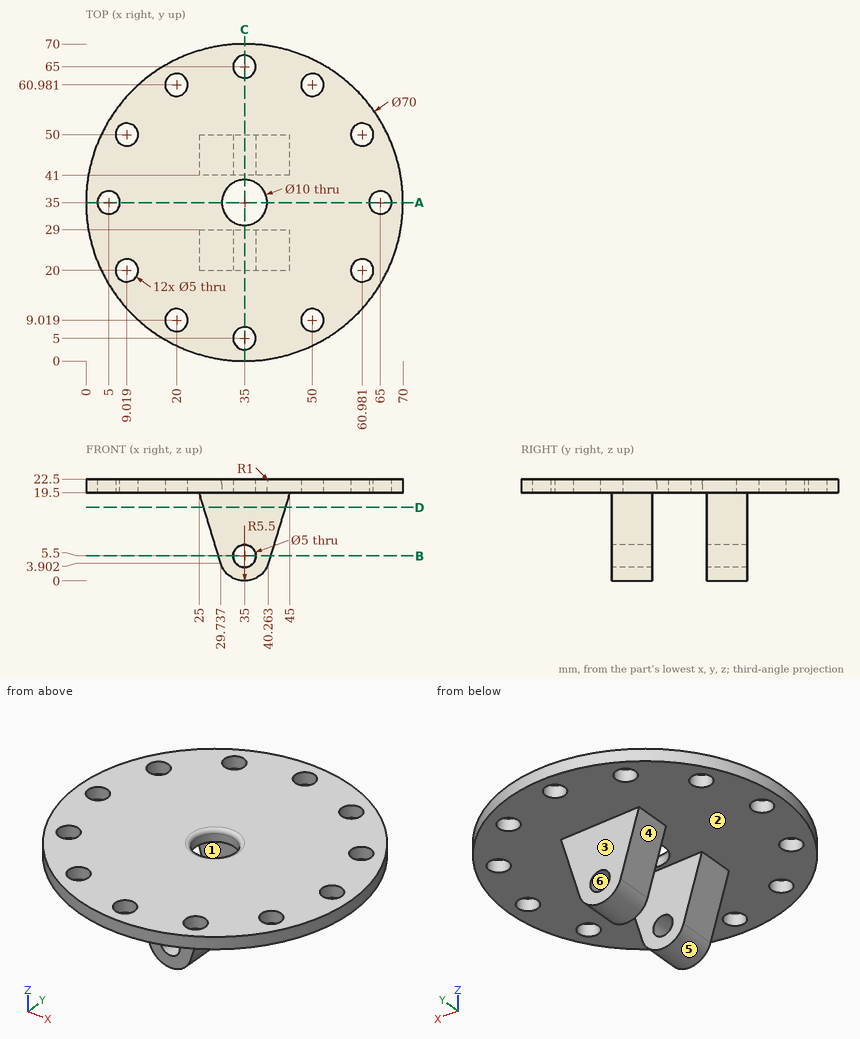
Study the drawing (mm; zero at the part's minimum x, y, z) and answer. A direction names the side the tool comes from. Give positions to 0.01 mm unless a question says otherwise; leave off trailing zeros. Write each loop counter-clockwise with the first axis right and the second up, starting at its lowest first coordinate (ties: lowest second). Pieces come first, ordered by that corner, then holes. Notation, with made-up numbers: (23.5, 3) - (48.5, 3) arc R18 cw to (48.5, 18) - close; hole circle Ø2 at (-17.5, 11.5). An arc over 180 degrees is marked (long way). Use CSV: the item, a comma, the result in double quotes. Start each with the question number.
(1) Given P1, Ø10, axis at x = 36, z = 7, coming from the +Y side; P2, Ø10, axis at x = 14, y = 62.5, coming from the -Z side; P3, Ø8, axis at x = 35, z = 5.5, coming from the -Y side; P4, Ø6, axis at x = 50, y = 9.02, coming from the +Z side, each flat-ended and moving along its own axis, determine where each tip first touches the part or whether it passes through.
(2) Find section B-B (z = 5.5). Give the vertices of the cut face in (x, y).
(3) Consider line 1 along Y through (x, z) = (35, 21.05); line 2 along Y through (x, z) = (34, 17); line 3 along Z through (x, y) = (36, 12). Determine where each line is inside the solid, lowest interval first.
(4) Find section D-D (z = 16.25). Give the vertices of the cut face in (x, y).
(5) For the marked faces 1, 2 and 3, determine the directions among +Z, -Z, +X, -X, +Y, -Y from which every point of the face is accessible in a straight line to the end or side of a thin tool.
(6) Find section A-A (y = 35). Give the vertices of the cut face in (x, z).
(7) Determine the mould class of the marked faces 4, 5 and 6 for opening direction X: +X half, -X half, draft (parallel to the pull), parting line (faces both ways), or undercut.
(8) Find section C-C (x = 35). Count the separate pieces of the cut face and the enclosed holes in it.
Findings below:
1,P1,"y = 50"
1,P2,"z = 19.5"
1,P3,"y = 20"
1,P4,"z = 22.5"
2,outline,"(29.25, 20) - (32.5, 20) - (32.5, 29) - (29.25, 29) - close; (29.25, 41) - (32.5, 41) - (32.5, 50) - (29.25, 50) - close; (37.5, 20) - (40.75, 20) - (40.75, 29) - (37.5, 29) - close; (37.5, 41) - (40.75, 41) - (40.75, 50) - (37.5, 50) - close"
3,line 1,"0 to 2.5, 7.5 to 30, 40 to 62.5, 67.5 to 70"
3,line 2,"20 to 29, 41 to 50"
3,line 3,"19.5 to 22.5"
4,outline,"(25.99, 20) - (44.01, 20) - (44.01, 29) - (25.99, 29) - close; (25.99, 41) - (44.01, 41) - (44.01, 50) - (25.99, 50) - close"
5,face 1,"-Z, +X, -X"
5,face 2,"-Z"
5,face 3,"-Z, +X, -X, +Y"
6,outline,"(0, 19.5) - (2.5, 19.5) - (2.5, 22.5) - (0, 22.5) - close; (7.5, 19.5) - (30, 19.5) - (30, 21.5) arc R1 ccw to (29, 22.5) - (7.5, 22.5) - close; (40, 19.5) - (62.5, 19.5) - (62.5, 22.5) - (41, 22.5) arc R1 ccw to (40, 21.5) - close; (67.5, 19.5) - (70, 19.5) - (70, 22.5) - (67.5, 22.5) - close"
7,face 4,"-X half"
7,face 5,"parting line"
7,face 6,"undercut"
8,separate pieces,"6"
8,enclosed holes,"0"
